```python
from build123d import *

# Parameters (mm, degrees)
BOSS_EXTRUDE1_DEPTH = 60
CUT_EXTRUDE1_REACH  = 3.5
SKETCH2_R           = 14
SKETCH2_R_2         = 2.5
CUT_EXTRUDE2_REACH  = 3.5
SKETCH3_R           = 1.5


with BuildPart() as part:
    # Sketch1 → Boss-Extrude1 (new body)
    with BuildSketch(Plane.XY):
        Polygon((0, 0), (0, 50), (1.5, 50), (1.5, 1.5), (190, 1.5), (190, 0), align=None)
    extrude(amount=BOSS_EXTRUDE1_DEPTH)

    # Sketch2 → Cut-Extrude1 (cut, up to next)
    with BuildSketch(Plane(origin=(1.5, 0, 0), x_dir=(0, 0, -1), z_dir=(1, 0, 0)), mode=Mode.PRIVATE) as cut_extrude1_sk1:
        with Locations((-30, 25)):
            Circle(SKETCH2_R)
    cut_extrude1_tool1 = extrude(cut_extrude1_sk1.sketch, amount=-CUT_EXTRUDE1_REACH, mode=Mode.PRIVATE) & part.part
    add(cut_extrude1_tool1.solids().sort_by_distance((1.5, 25, 30))[0], mode=Mode.SUBTRACT)
    # Sketch2 → Cut-Extrude1 (cut, up to next)
    with BuildSketch(Plane(origin=(1.5, 0, 0), x_dir=(0, 0, -1), z_dir=(1, 0, 0)), mode=Mode.PRIVATE) as cut_extrude1_sk2:
        with Locations((-55, 25)):
            Circle(SKETCH2_R_2)
    cut_extrude1_tool2 = extrude(cut_extrude1_sk2.sketch, amount=-CUT_EXTRUDE1_REACH, mode=Mode.PRIVATE) & part.part
    add(cut_extrude1_tool2.solids().sort_by_distance((1.5, 25, 55))[0], mode=Mode.SUBTRACT)
    # Sketch2 → Cut-Extrude1 (cut, up to next)
    with BuildSketch(Plane(origin=(1.5, 0, 0), x_dir=(0, 0, -1), z_dir=(1, 0, 0)), mode=Mode.PRIVATE) as cut_extrude1_sk3:
        with Locations((-5, 25)):
            Circle(SKETCH2_R_2)
    cut_extrude1_tool3 = extrude(cut_extrude1_sk3.sketch, amount=-CUT_EXTRUDE1_REACH, mode=Mode.PRIVATE) & part.part
    add(cut_extrude1_tool3.solids().sort_by_distance((1.5, 25, 5))[0], mode=Mode.SUBTRACT)

    # Sketch3 → Cut-Extrude2 (cut, up to next)
    with BuildSketch(Plane(origin=(0, 1.5, 0), x_dir=(1, 0, 0), z_dir=(0, 1, 0)), mode=Mode.PRIVATE) as cut_extrude2_sk1:
        with Locations((160, -11)):
            Circle(SKETCH3_R)
    cut_extrude2_tool1 = extrude(cut_extrude2_sk1.sketch, amount=-CUT_EXTRUDE2_REACH, mode=Mode.PRIVATE) & part.part
    add(cut_extrude2_tool1.solids().sort_by_distance((160, 1.5, 11))[0], mode=Mode.SUBTRACT)
    # Sketch3 → Cut-Extrude2 (cut, up to next)
    with BuildSketch(Plane(origin=(0, 1.5, 0), x_dir=(1, 0, 0), z_dir=(0, 1, 0)), mode=Mode.PRIVATE) as cut_extrude2_sk2:
        with Locations((176, -11)):
            Circle(SKETCH3_R)
    cut_extrude2_tool2 = extrude(cut_extrude2_sk2.sketch, amount=-CUT_EXTRUDE2_REACH, mode=Mode.PRIVATE) & part.part
    add(cut_extrude2_tool2.solids().sort_by_distance((176, 1.5, 11))[0], mode=Mode.SUBTRACT)
    # Sketch3 → Cut-Extrude2 (cut, up to next)
    with BuildSketch(Plane(origin=(0, 1.5, 0), x_dir=(1, 0, 0), z_dir=(0, 1, 0)), mode=Mode.PRIVATE) as cut_extrude2_sk3:
        with Locations((176, -49)):
            Circle(SKETCH3_R)
    cut_extrude2_tool3 = extrude(cut_extrude2_sk3.sketch, amount=-CUT_EXTRUDE2_REACH, mode=Mode.PRIVATE) & part.part
    add(cut_extrude2_tool3.solids().sort_by_distance((176, 1.5, 49))[0], mode=Mode.SUBTRACT)
    # Sketch3 → Cut-Extrude2 (cut, up to next)
    with BuildSketch(Plane(origin=(0, 1.5, 0), x_dir=(1, 0, 0), z_dir=(0, 1, 0)), mode=Mode.PRIVATE) as cut_extrude2_sk4:
        with Locations((160, -49)):
            Circle(SKETCH3_R)
    cut_extrude2_tool4 = extrude(cut_extrude2_sk4.sketch, amount=-CUT_EXTRUDE2_REACH, mode=Mode.PRIVATE) & part.part
    add(cut_extrude2_tool4.solids().sort_by_distance((160, 1.5, 49))[0], mode=Mode.SUBTRACT)


solid = part.part
```
Verification items for the finished model (mm, model axes). A direction names the side the tool comes from. Coordinates: 2 decimals unless noted, no trailing zeros. Loops run counter-clockwise (first coordinate to the right, second up) from the corner with the lowest first, then second, coordinate; pieces in that order, holes last. Notation, with made-up numbers: (33.5, 20.5) -> (78.5, 20.5) arc R25 cw to (78.5, 59.5) -> close; hole circle Ø4 at (65, -23). An arc over 180 degrees is marked (long way). Answer in a Markdown table with one row per item.
1) Section check A-A (z = 5). Record the cut outline in (x, y).
The answers:
| item | result |
|---|---|
| outline | (0, 0) -> (190, 0) -> (190, 1.5) -> (1.5, 1.5) -> (1.5, 22.5) -> (0, 22.5) -> close; (0, 27.5) -> (1.5, 27.5) -> (1.5, 50) -> (0, 50) -> close |
2) Scan lines: line 1 along X through (y, z) = (1.05, 11); line 2 along Z through (x, y) = (176, 1); line 3 along Y through (x, z) = (1, 5). Record each from-to range of solid material in increasing order. Write a range as from..to.
The answers:
| item | result |
|---|---|
| line 1 | x = 0..158.5, 161.5..174.5, 177.5..190 |
| line 2 | z = 0..9.5, 12.5..47.5, 50.5..60 |
| line 3 | y = 0..22.5, 27.5..50 |
3) Section check B-B (z = 30). Record the cut outline in (x, y).
The answers:
| item | result |
|---|---|
| outline | (0, 0) -> (190, 0) -> (190, 1.5) -> (1.5, 1.5) -> (1.5, 11) -> (0, 11) -> close; (0, 39) -> (1.5, 39) -> (1.5, 50) -> (0, 50) -> close |
4) Depth check by flat-ended pin: P1, Ø1.8, axis at x = 160, z = 49, coming from the +Y side; P2, Ø8, axis at x = 116, z = 29, coming from the +Y side. Enter the tip coordinate at first touch or a pass-through.
The answers:
| item | result |
|---|---|
| P1 | passes through |
| P2 | stops at y = 1.5 |
5) Section check C-C (y = 8.5). Record the cut outline in (x, z).
The answers:
| item | result |
|---|---|
| outline | (0, 0) -> (1.5, 0) -> (1.5, 60) -> (0, 60) -> close |
6) Access from +Z, -Z, +X, -X, +Y, -Y to the whole of each face (thin tool, end or side, straight path). Record for faces 4 (the face through (0.76, 27.11, 53.66)), 5 (the face through (1.5, 31, 16)).
The answers:
| item | result |
|---|---|
| face 4 | +X, -X |
| face 5 | +Z, -Z, +X, +Y |
7) Draft check along Y on faces 1 (the face through (96, 0, 30)), 2 (the face through (0.76, 25.616, 43.986)), 3 (the face through (0, 19, 16)). Enter one of: released by +Y, released by -Y, zero draft, split by the parting line, or undercut.
The answers:
| item | result |
|---|---|
| face 1 | released by -Y |
| face 2 | undercut |
| face 3 | zero draft |
